Check sheet for the modelled part. Datum: model origin and axes. Units: mm. A direction names the side the tool comes from. Give positions to 0.01 mm unless a question says otherwise; leave off trailing zeros. Write each loop counter-clockwise with the first axis right and the second up, starting at its lowest first coordinate (ties: lowest second). Pieces come first, ordered by that corner, then holes. Notation, with made-up numbers: M 62,-36 L 114,-36 A26 cw 114,-20 Z; hole C 27.5,42 d2. An arc over 180 degrees is marked long. One line per item, written item: value. Start each with the question number.
from build123d import *

# Parameters (mm, degrees)
F1_DEPTH = 50.8
F2_R     = 4.7625
F3_DEPTH = 60.325


with BuildPart() as f1:
    # F0 (on Top) → F1 (new body, symmetric)
    with BuildSketch(Plane.XY):
        Polygon((31.75, -18.330871), (0, 36.661742), (-31.75, -18.330871), align=None)
    extrude(amount=F1_DEPTH, both=True)

    # F2 (on Top) → F3 (join, symmetric)
    with BuildSketch(Plane.XY):
        Circle(F2_R)
    extrude(amount=F3_DEPTH, both=True)


solid = f1.part
1) Gauge pin test, flat ends, axial feed: pin 1 (1.5 mm diameter, centred on y = 18, z = -40.5, fed in from -X); pin 2 (8 mm diameter, centred on y = 0.5, z = -16, fed in from +X); pin 3 (10 mm diameter, centred on y = -9.5, z = 2, fed in from +X). Record the tip position at first contact, or that the pin passes through.
2) Cross-section at A-A (y = 0). Record the boundary of the cut face in (x, z) (1 decimal).
3) Cross-section at B-B (z = -17). Record the boundary of the cut face in (x, y), plus the area to 3 significant figures.
4) Cross-section at C-C (x = -19.5). Record the boundary of the cut face in (y, z), plus the area to 3 significant figures.
5) Cross-section at D-D (y = 27.5). Record the boundary of the cut face in (x, z).
6) Material ranges on L1, parallel to Z at x = -14.5, y = -11; L2, parallel to Y at x = 1.5, z = 28.5; L3, parallel to X at y = 26, z = 6, recorded low to high. Write a range as from..to.
7) Tool access check on faces 1 (the cylindrical face through (-3.78, -2.9, -55.5)), 2 (the flat face through (0, 0, -60.325)), 3 (the cylindrical face through (-3.78, -2.9, 55.63)). Record the directions out of +Z, -Z, +X, -X, +Y, -Y that give a thin tool (end or side, any length) a straight path to the whole face; none if there is none.
Data:
1. pin 1: stops at x = -11.21
1. pin 2: stops at x = 23.19
1. pin 3: stops at x = 29.54
2. outline: M -21.2,-50.8 L -4.8,-50.8 L -4.8,-60.3 L 4.8,-60.3 L 4.8,-50.8 L 21.2,-50.8 L 21.2,50.8 L 4.8,50.8 L 4.8,60.3 L -4.8,60.3 L -4.8,50.8 L -21.2,50.8 Z
3. outline: M -31.75,-18.33 L 31.75,-18.33 L 0,36.66 Z
3. area: 1,750 mm2
4. outline: M -18.33,-50.8 L 2.89,-50.8 L 2.89,50.8 L -18.33,50.8 Z
4. area: 2,160 mm2
5. outline: M -5.29,-50.8 L 5.29,-50.8 L 5.29,50.8 L -5.29,50.8 Z
6. L1: z = -50.8..50.8
6. L2: y = -18.33..34.06
6. L3: x = -6.16..6.16
7. face 1: -Z
7. face 2: -Z, +X, -X, +Y, -Y
7. face 3: +Z
